Read the model definition and answer for the solid it produces. Units are mm, in the model's axes. A direction names the side the tool comes from. Round coordinates to 2 decimals unless told otherwise and drop trailing zeros. Loops run counter-clockwise (first coordinate to the right, second up) from the corner with the lowest first, then second, coordinate; pieces in that order, holes last. Notation, with made-up numbers: M 89.25,-30 L 113.25,-30 A26 cw 113.25,0 Z; hole C 80.5,-28.5 d4. An arc over 180 degrees is marked long. Answer as CSV lines item,"result".
```python
from build123d import *

# Parameters (mm, degrees)
BOSS_EXTRUDE1_DEPTH = 63.5
SKETCH3_W           = 52.197
SKETCH3_H           = 52.197
BOSS_EXTRUDE2_DEPTH = 20.574
SKETCH_D_R          = 14.2875
BOSS_EXTRUDE3_DEPTH = 63.5
CUT_EXTRUDE1_DEPTH  = 35.56
FILLET1_R           = 6.35
FILLET2_R           = 1.27
KEYWAY_START        = 10.7569
KEYWAY_DEPTH        = 47.3931
CHAMFER1_SIZE       = 0.381
SKETCH7_R           = 14.2875
CUT_EXTRUDE3_DEPTH  = 148.574


with BuildPart() as part:
    # L,M → Boss-Extrude1 (new body)
    with BuildSketch(Plane.XY):
        Polygon((-66.675, 53.975), (66.675, 53.975), (66.675, 151.07969491), (52.451, 165.30369491), (52.451, 212.64830509), (18.97330509, 246.126), (-18.97330509, 246.126), (-52.451, 212.64830509), (-52.451, 165.30369491), (-66.675, 151.07969491), align=None)
    extrude(amount=BOSS_EXTRUDE1_DEPTH)

    # Sketch3 → Boss-Extrude2 (add)
    with BuildSketch(Plane.XY.offset(63.5)):
        with Locations((0, 188.976)):
            Rectangle(SKETCH3_W, SKETCH3_H)
    extrude(amount=BOSS_EXTRUDE2_DEPTH)

    # D → Boss-Extrude3 (add)
    with BuildSketch(Plane.XY.offset(84.074)):
        with Locations((0, 188.976)):
            Circle(SKETCH_D_R)
    extrude(amount=BOSS_EXTRUDE3_DEPTH)

    # Sketch5 → Cut-Extrude1 (cut)
    with BuildSketch(Plane.XY.offset(63.5)):
        Polygon((66.675, 87.45269491), (33.19730509, 53.975), (66.675, 53.975), align=None)
        Polygon((-66.675, 53.975), (-66.675, 87.45269491), (-33.19730509, 53.975), align=None)
    extrude(amount=-CUT_EXTRUDE1_DEPTH, mode=Mode.SUBTRACT)

    # Fillet1
    fillet1_edges = [part.edges().sort_by_distance(p)[0] for p in [
        (-26.0985, 215.0745, 73.787),
        (-26.0985, 162.8775, 73.787),
        (26.0985, 162.8775, 73.787),
        (26.0985, 215.0745, 73.787),
    ]]
    fillet(fillet1_edges, radius=FILLET1_R)

    # Fillet2
    fillet2_edges = [part.edges().sort_by_distance(p)[0] for p in [
        (66.675, 119.26619491, 63.5),
        (49.936152545, 70.713847455, 63.5),
        (59.563, 158.19169491, 63.5),
        (52.451, 188.976, 63.5),
        (35.712152545, 229.387152545, 63.5),
        (0, 53.975, 63.5),
        (0, 246.126, 63.5),
        (-35.712152545, 229.387152545, 63.5),
        (-52.451, 188.976, 63.5),
        (-59.563, 158.19169491, 63.5),
        (-66.675, 119.26619491, 63.5),
        (-49.936152545, 70.713847455, 63.5),
        (0, 162.8775, 63.5),
        (-26.0985, 188.976, 63.5),
        (26.0985, 188.976, 63.5),
        (0, 215.0745, 63.5),
        (-24.238628061, 164.737371939, 63.5),
        (24.238628061, 164.737371939, 63.5),
        (-24.238628061, 213.214628061, 63.5),
        (24.238628061, 213.214628061, 63.5),
    ]]
    fillet(fillet2_edges, radius=FILLET2_R)

    # Sketch6 → Keyway (cut, through all)
    with BuildSketch(Plane(origin=(0, 188.976, 0), x_dir=(-1, 0, 0), z_dir=(0, 1, 0)).offset(KEYWAY_START)):
        with BuildLine():
            Line((3.175, 147.574), (3.175, 89.154))
            ThreePointArc((3.175, 89.154), (0, 85.979), (-3.175, 89.154))
            Line((-3.175, 89.154), (-3.175, 147.574))
            ThreePointArc((-3.175, 147.574), (0, 150.749), (3.175, 147.574))
        make_face()
    extrude(amount=KEYWAY_DEPTH, mode=Mode.SUBTRACT)

    # Chamfer1
    chamfer1_edges = [part.edges().sort_by_distance(p)[0] for p in [
        (-8.909821652, 177.806947472, 147.574),
    ]]
    chamfer(chamfer1_edges, length=CHAMFER1_SIZE)

    # Sketch7 → Cut-Extrude3 (cut, through all)
    with BuildSketch(Plane(origin=(0, 0, 0), x_dir=(-1, 0, 0), z_dir=(0, 0, -1))):
        with Locations((0, 107.95)):
            Circle(SKETCH7_R)
    extrude(amount=-CUT_EXTRUDE3_DEPTH, mode=Mode.SUBTRACT)


solid = part.part
```
1) Determine the mould class of faces 5 (the flat face through (0, 162.878, 74)), 6 (the cylindrical face through (24.2, 164.7, 74.6)), 7 (the cylindrical face through (1.86, 122.116, 31.306)) for opening direction X: released by +X, released by -X, zero draft, split by the parting line, or undercut.
Evaluation:
face 5,"zero draft"
face 6,"released by +X"
face 7,"undercut"
2) A tool of negligible diameter and unlimited length cuts with its end or side. For faces 1 (the cylindrical face through (24.29, 213.16, 74.56)), 2 (the flat face through (-12, 178, 84.074)), 3 (the flat face through (52.451, 189, 31)), 4 (the flat face through (26.098, 189, 74)), from which of +Z, -Z, +X, -X, +Y, -Y can it reach the whole face along a straight path? Write none if from no direction.
Evaluation:
face 1,"+Z, +X, +Y"
face 2,"+Z"
face 3,"+Z, -Z, +X, +Y"
face 4,"+Z, +X, +Y, -Y"
3) Find section A-A, the plane y = 107.95. Give the vertices of the cut face in (x, z) (1 decimal).
Evaluation:
outline,"M -66.7,0 L -14.3,0 L -14.3,63.5 L -65.4,63.5 A1.3 ccw -66.7,62.2 Z; M 14.3,0 L 66.7,0 L 66.7,62.2 A1.3 ccw 65.4,63.5 L 14.3,63.5 Z"
4) Straight lines are drawn through the part: line 1 (Y direction, x = 0, z = 44) (1 decimal); line 2 (X direction, y = 107, z = 36) (3 decimals); line 3 (Z direction, x = -21, y = 171.5). For each, find the intervals that lie inside material, in ascending order.
Evaluation:
line 1,"y = 54 to 93.7, 122.2 to 246.1"
line 2,"x = -66.675 to -14.256, 14.256 to 66.675"
line 3,"z = 0 to 84.07"
5) Each of these flat-tipped pins is pushed along its axis until it touches: P1, Ø10, axis at x = 45.5, y = 179.5, coming from the -Z side; P2, Ø8, axis at x = 36, z = 57, coming from the +Y side; P3, Ø12, axis at y = 168, z = 22, coming from the -X side; P4, Ø6, axis at x = 3.5, z = 71.5, coming from the +Y side. Where does it stop, or does it pass through?
Evaluation:
P1,"stops at z = 0"
P2,"stops at y = 233.1"
P3,"stops at x = -55.75"
P4,"stops at y = 215.07"
6) Find section C-C, the plane x = 0. Give the vertices of the cut face in (y, z) (1 decimal).
Evaluation:
outline,"M 54,0 L 93.7,0 L 93.7,63.5 L 55.2,63.5 A1.3 ccw 54,62.2 Z; M 122.2,0 L 246.1,0 L 246.1,62.2 A1.3 ccw 244.9,63.5 L 216.3,63.5 A1.3 cw 215.1,64.8 L 215.1,84.1 L 203.3,84.1 L 203.3,86 L 199.7,86 L 199.7,147.6 L 175.1,147.6 L 174.7,147.2 L 174.7,84.1 L 162.9,84.1 L 162.9,64.8 A1.3 cw 161.6,63.5 L 122.2,63.5 Z"
7) Find section D-D, the plane z = 78. Give the vertices of the cut face in (x, y), then the cut area to 3 significant figures.
Evaluation:
outline,"M -26.1,169.23 A6.35 ccw -19.75,162.88 L 19.75,162.88 A6.35 ccw 26.1,169.23 L 26.1,208.72 A6.35 ccw 19.75,215.07 L -19.75,215.07 A6.35 ccw -26.1,208.72 Z"
area,"2,690 mm^2"
